from build123d import *

# Parameters (mm, degrees)
F0_W     = 31.75
F0_H     = 25.4
F1_DEPTH = 12.7
F2_W     = 29.718
F2_H     = 24.13
F3_DEPTH = 2.54
F4_W     = 29.718
F4_H     = 24.13
F4_W_2   = 25.908
F4_H_2   = 20.32
F5_DEPTH = 10.16
F5_TAPER = 1
F6_W     = 31.75
F6_H     = 25.4
F7_DEPTH = 2.54


with BuildPart() as f1:
    # F0 (on Top) → F1 (new body)
    with BuildSketch(Plane.XY):
        with Locations((-15.875, -12.7)):
            Rectangle(F0_W, F0_H)
    extrude(amount=F1_DEPTH)

    # F2 (on face) → F3 (cut)
    with BuildSketch(Plane.XY.offset(12.7)):
        with Locations((-15.875, -12.7)):
            Rectangle(F2_W, F2_H)
    extrude(amount=-F3_DEPTH, mode=Mode.SUBTRACT)

    # F4 (on face) → F5 (cut)
    with BuildSketch(Plane.XY.offset(10.16)):
        with Locations((-15.875, -12.7)):
            Rectangle(F4_W, F4_H)
        with Locations((-15.875, -12.7)):
            Rectangle(F4_W_2, F4_H_2, mode=Mode.SUBTRACT)
    extrude(amount=-F5_DEPTH, taper=F5_TAPER, mode=Mode.SUBTRACT)

    # F6 (on face) → F7 (join)
    with BuildSketch(Plane(origin=(0, 0, 0), x_dir=(1, 0, 0), z_dir=(0, 0, -1))):
        with Locations((-15.875, 12.7)):
            Rectangle(F6_W, F6_H)
    extrude(amount=F7_DEPTH)


solid = f1.part
Source: CAD feature listing. Evaluate the final solid. Frame: model axes, mm. A direction names the side the tool comes from. Coordinates: 2 decimals unless noted, no trailing zeros. Loops run counter-clockwise (first coordinate to the right, second up) from the corner with the lowest first, then second, coordinate; pieces in that order, holes last. Notation, with made-up numbers: (-15.5, 52) - (6.5, 52) arc R19 cw to (6.5, 75) - close; hole circle Ø11 at (22.5, -4.5). An arc over 180 degrees is marked (long way). Return JSON: item names as keys, results as strings.
Q1. Section A-A, the plane z = 10.75. Return loops of the section in (x, y) (3 decimals), plus the area to 3 significant figures.
Results:
{"outline": "(-31.75, -25.4) - (0, -25.4) - (0, 0) - (-31.75, 0) - close; hole (-30.734, -24.765) - (-1.016, -24.765) - (-1.016, -0.635) - (-30.734, -0.635) - close", "area": "89.4 mm2"}
Q2. Access query for faces 4 (the flat face through (-16, -24.765, 11)), 5 (the flat face through (-16, -13, -2.54)). Directions: +Z, -Z, +X, -X, +Y, -Y. A direction counts if a zero-diameter tool reaches every point of the face in a straight line with its end or side. Return the directions, or none.
Results:
{"face 4": "+Z", "face 5": "-Z, +X, -X, +Y, -Y"}
Q3. Section B-B, the plane z = 2. Give the number of separate pieces and of enclosed holes in the cut face, plus the area to 3 significant figures.
Results:
{"separate pieces": "2", "enclosed holes": "1", "area": "644 mm2"}
Q4. Contact query for a flat-ended pin moving along its axis: P1, Ø3, axis at x = -23, y = -11.5, coming from the +Z side. Output: stop coordinate, or through.
Results:
{"P1": "z = 10.16"}
Q5. Material intervals for line 1 along Y through (x, z) = (-16.5, 0.5); line 2 along Y through (x, z) = (-22, 11.25) (3 decimals); line 3 along X through (y, z) = (-15.5, 1), sorted ascending.
Results:
{"line 1": "-25.4 to -24.6, -23.03 to -2.37, -0.8 to 0", "line 2": "-25.4 to -24.765, -0.635 to 0", "line 3": "-31.75 to -30.57, -28.99 to -2.76, -1.18 to 0"}
Q6. Mould query, pull axis X, two halves, no side actions, for faces 1 (the flat face through (-16, 0, 5)), 2 (the flat face through (-1.016, -13, 11)), 3 (the flat face through (-31.75, -13, 5)). Classes: released by +X, released by -X, zero draft, split by the parting line, or undercut.
Results:
{"face 1": "zero draft", "face 2": "undercut", "face 3": "released by -X"}
